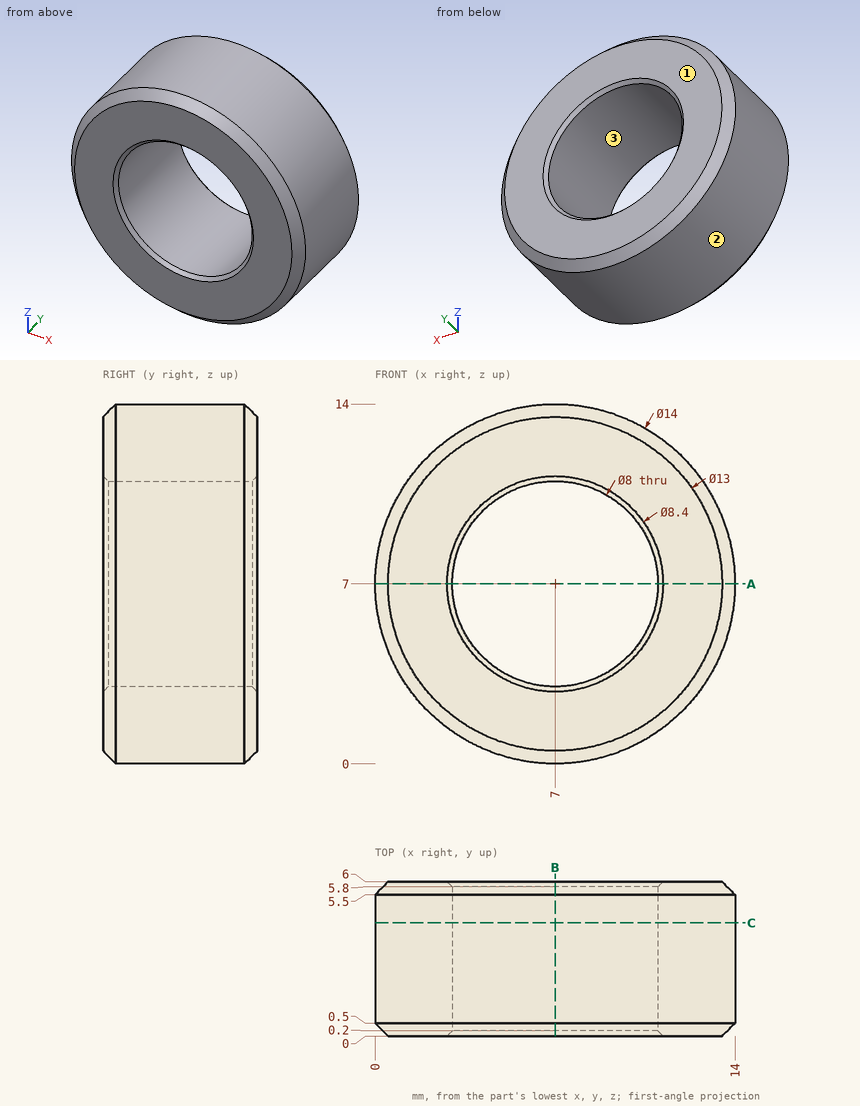
Job drawing, mm, ordinate dimensions from the low corner. One solid piece. Coordinates: 2 decimals unless noted, no trailing zeros. Write each loop counter-clockwise with the first axis right and the second up, starting at its lowest first coordinate (ties: lowest second). Pieces come first, ordered by that corner, then holes. Notation, with made-up numbers: M 39,-10.75 L 61,-10.75 A16 cw 61,-6.75 Z; hole C 65.5,50 d6. An arc over 180 degrees is marked long. Answer as a JSON object with one key per item and string values. Group by question number.
1) Pin check, flat tip, straight feed: pin 1 Ø1 at (x, y) = (8.5, 1) entering from -Z. Stop position of the tip, or through.
2) Wall check: line 1 (X direction, y = 4.45, z = 7); line 2 (X direction, y = 2.15, z = 6); line 3 (Z direction, x = 4, y = 5.3). Give the ranges that are in metal, low to high. Write a range as from..to.
3) Mould opens along Z. For the marked faces 1, 2 and 3 say: +Z half, -Z half, draft (parallel to the pull), parting line (faces both ways), or undercut.
4) Saw through at B-B (x = 7). Write the cut outline in (y, z), plus the area to 3 significant figures.
5) Saw through at C-C (y = 4.4). Write the cut outline in (x, z).
6) Saw through at A-A (z = 7). Write the cut outline in (x, y).
Values follow:
{
 "1": {"pin 1": "stops at z = 0.07"},
 "2": {"line 1": "x = 0..3, 11..14", "line 2": "x = 0.07..3.13, 10.87..13.93", "line 3": "z = 0.68..4.35, 9.65..13.32"},
 "3": {"face 1": "draft", "face 2": "parting line", "face 3": "undercut"},
 "4": {"outline": "M 0,0.5 L 0.5,0 L 5.5,0 L 6,0.5 L 6,2.8 L 5.8,3 L 0.2,3 L 0,2.8 Z; M 0,11.2 L 0.2,11 L 5.8,11 L 6,11.2 L 6,13.5 L 5.5,14 L 0.5,14 L 0,13.5 Z", "area": "35.4 mm2"},
 "5": {"outline": "C 7,7 d14; hole C 7,7 d8"},
 "6": {"outline": "M 0,0.5 L 0.5,0 L 2.8,0 L 3,0.2 L 3,5.8 L 2.8,6 L 0.5,6 L 0,5.5 Z; M 11,0.2 L 11.2,0 L 13.5,0 L 14,0.5 L 14,5.5 L 13.5,6 L 11.2,6 L 11,5.8 Z"}
}
